Source: three-view drawing plus pictorial views. Frame: mm from the lowest corner of the part. A direction names the side the tool comes from. Round coordinates to 2 decimals unless told otherwise and drop trailing zeros. Loops run counter-clockwise (first coordinate to the right, second up) from the corner with the lowest first, then second, coordinate; pieces in that order, holes last. Notation, with made-up numbers: (37, 71) -> (94, 71) arc R23 cw to (94, 109) -> close; hole circle Ø3 at (-21.75, -21.75). An arc over 180 degrees is marked (long way). Answer in a Markdown table with one row per item. Add a question column.
Q1. Section B-B, the plane z = 7.75. Output: boundary loops of the cut face in (x, y), and give its area (3 significant figures).
Q2. Pin query (flat end, axial travel): pin 1 (1 mm diameter, centred on x = 7, y = 8, fed in from +Z); pin 2 (1 mm diameter, centred on y = 9.5, z = 3, fed in from -X). Return the tip coordinate at first contact, or that it passes through.
Q3. Section D-D, the plane z = 0.75. Output: boundary loops of the cut face in (x, y), and give its area (3 significant figures).
Q4. Reachability of the marked faces 1 and 2 from +Z, -Z, +X, -X, +Y, -Y: full face, straight path, thin tool, end or side. Return the list, or none.
Q5. Section A-A, the plane x = 7.5. Output: boundary loops of the cut face in (y, z).
Q6. Ray query, L1, parallel to Y at x = 7.5, z = 4.25; L2, parallel to Z at x = 6.75, y = 13.5; L3, parallel to Y at x = 8, z = 3.25. Return the intervals inside material, ascending. Write a range as from..to.
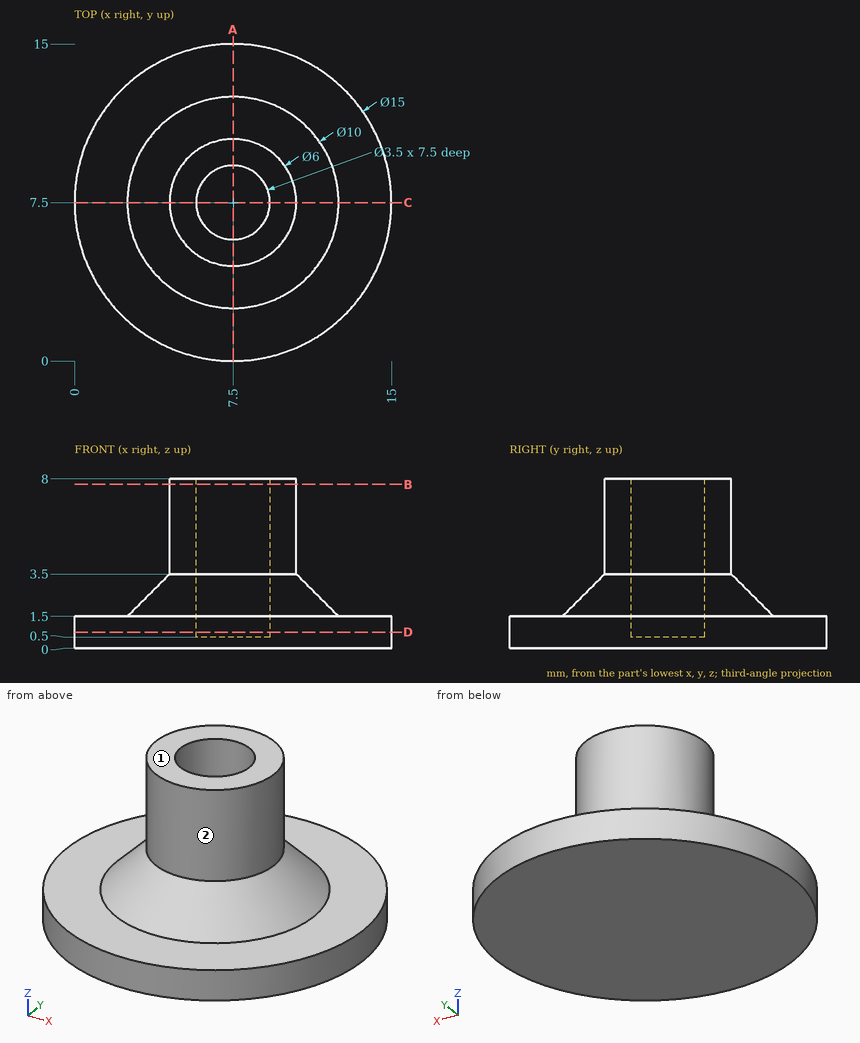
Answer block:
| question | item | result |
|---|---|---|
| 1 | outline | circle Ø6 at (7.5, 7.5); hole circle Ø3.5 at (7.5, 7.5) |
| 1 | area | 18.7 mm^2 |
| 2 | pin 1 | z = 0.5 |
| 2 | pin 2 | x = 3.97 |
| 3 | outline | circle Ø15 at (7.5, 7.5); hole circle Ø3.5 at (7.5, 7.5) |
| 3 | area | 167 mm^2 |
| 4 | face 1 | +Z, +X, -X, +Y, -Y |
| 4 | face 2 | +Z |
| 5 | outline | (0, 0) -> (15, 0) -> (15, 1.5) -> (12.5, 1.5) -> (10.5, 3.5) -> (10.5, 8) -> (9.25, 8) -> (9.25, 0.5) -> (5.75, 0.5) -> (5.75, 8) -> (4.5, 8) -> (4.5, 3.5) -> (2.5, 1.5) -> (0, 1.5) -> close |
| 6 | L1 | 4.5..5.75, 9.25..10.5 |
| 6 | L2 | 0..1.5 |
| 6 | L3 | 4.29..5.82, 9.18..10.71 |
